Autodesk Inventor part; units mm, degrees
ref_plane "YZ Plane" through (0, 0, 0) normal (1, 0, 0) x (0, 1, 0)
ref_plane "XZ Plane" through (0, 0, 0) normal (0, 1, 0) x (-1, 0, 0)
ref_plane "XY Plane" through (0, 0, 0) normal (0, 0, 1) x (1, 0, 0)
sketch "Sketch1" plane through (0, 0, 0) normal (0, 0, 1) x (1, 0, 0)
  line L0 (-4.1767, 5.9085) -> (6.2233, 5.9085)
  line L1 (6.2233, 5.9085) -> (6.2233, -7.1915)
  line L2 (6.2233, -7.1915) -> (-4.1767, -7.1915)
  line L3 (-4.1767, -7.1915) -> (-4.1767, 5.9085)
  point P0 (0, 0)
  dimension "d0" = 10.4
  dimension "d1" = 13.1
extrude "Extrusion1" add sketch "Sketch1" along normal blind 2
sketch "Sketch2" plane through (0, 0, 2) normal (0, 0, 1) x (1, 0, 0)
  line L0 (-4.1767, -7.1915) -> (6.2233, -7.1915)
  line L1 (6.2233, -7.1915) -> (6.2233, 5.9085)
  line L2 (6.2233, 5.9085) -> (-4.1767, 5.9085)
  line L3 (-4.1767, 5.9085) -> (-4.1767, -7.1915)
  line L4 (6.2233, 5.9085) -> (-4.1767, 5.9085)
  line L5 (1.0233, 5.9085) -> (1.0233, -7.1915)
  line L6 (-4.1767, -7.1915) -> (6.2233, -7.1915)
  line L7 (6.2233, -7.1915) -> (6.2233, 5.9085)
  line L8 (6.2233, -0.6415) -> (-4.1767, -0.6415)
  line L9 (-4.1767, 5.9085) -> (-4.1767, -7.1915)
  line L10 (1.0233, -5.4195) -> (-3.5655, -5.4195)
  line L11 (-3.5655, -5.4195) -> (-3.5655, -2.8116)
  line L12 (-3.5655, -2.8116) -> (1.0233, -2.8116)
  line L13 (1.0233, -2.8116) -> (1.0233, -5.4195)
  point P0 (0, 0)
extrude "Extrusion2" add sketch "Sketch2" along normal blind 1.5 contours L10 L11 L12 L5
sketch "Sketch3" plane through (-3.5655, -2.8116, 2) normal (0, 1, 0) x (1, 0, 0)
  line L0 (0, 0) -> (4.5888, 0)
  line L1 (0, 0) -> (0, -1.5)
  line L2 (4.5888, -1.5) -> (0, -1.5)
  line L3 (4.5888, 0) -> (4.5888, -1.5)
  line L4 (4.5888, -1.5) -> (0, -1.5)
  line L5 (0, 0) -> (0, -1.5)
  line L6 (0, -1.5) -> (-10.2377, -47.6792)
  line L7 (4.5888, -1.5) -> (14.8265, -47.6792)
  arc A0 (-10.2377, -47.6792) -> (14.8265, -47.6792) centre (2.2944, 8.8493) ccw
  line L8 (0, -1.5) -> (4.5888, -1.5)
  point P0 (3.5655, 2)
properties part number "tof"
Can you work these out from the model? Positions are in its coordinate system, mm. A direction names the side the tool comes from. Round coordinates to 2 decimals unless told otherwise and drop trailing zeros. Loops run counter-clockwise (first coordinate to the right, second up) from the corner with the lowest first, then second, coordinate; pieces in that order, holes last. Notation, with made-up numbers: (37, -30) - (41, -30) arc R15 cw to (41, -9) - close; hole circle Ø2 at (-36.5, 27). An arc over 180 degrees is marked (long way). Use CSV: the item, a comma, the result in double quotes. Start each with the question number.
1) If we section it at A-A on y = -5.25: Write out the boundary of the cut face in (x, z).
2) Please list where these lines run through material, in increasing order: probe 1 along Z at (x, y) = (4.5, 0.75); probe 2 along Y at (x, z) = (-2.25, 3.25); probe 3 along X at (y, z) = (-4.25, 2.1). Write a range as [from, to].
3) If we section it at B-B on x = -1.75: Write out the boundary of the cut face in (y, z).
4) For faces 1 (the flat face through (-1, -5.42, 3)), 2 (the flat face through (-4.177, -1, 1)), 3 (the flat face through (1.023, -4, 3)), 4 (the flat face through (-1, -2.812, 3)), 5 (the flat face through (-3.566, -4, 3)), which set-ups out of +Z, -Z, +X, -X, +Y, -Y let a thin tool reach every point of the face, with its end or its side?
5) If we section it at C-C on z = 2.7: Write out the boundary of the cut face in (x, y), plus the area to 3 significant figures.
6) If we section it at D-D on y = 2: Write out the boundary of the cut face in (x, z), plus the area to 3 significant figures.
7) For pin 1 Ø5 at (x, y) = (-0.5, 3.5) entering from +Z; pin 2 Ø0.8 at (y, z) = (-4, 2.5) entering from +X, each with a flat end and sliding along its axis, tell me the tip position at first contact or that it passes through.
Geometry results:
1,outline,"(-4.18, 0) - (6.22, 0) - (6.22, 2) - (1.02, 2) - (1.02, 3.5) - (-3.57, 3.5) - (-3.57, 2) - (-4.18, 2) - close"
2,probe 1,"z = [0, 2]"
2,probe 2,"y = [-5.42, -2.81]"
2,probe 3,"x = [-3.57, 1.02]"
3,outline,"(-7.19, 0) - (5.91, 0) - (5.91, 2) - (-2.81, 2) - (-2.81, 3.5) - (-5.42, 3.5) - (-5.42, 2) - (-7.19, 2) - close"
4,face 1,"+Z, +X, -X, -Y"
4,face 2,"+Z, -Z, -X, +Y, -Y"
4,face 3,"+Z, +X, +Y, -Y"
4,face 4,"+Z, +X, -X, +Y"
4,face 5,"+Z, -X, +Y, -Y"
5,outline,"(-3.57, -5.42) - (1.02, -5.42) - (1.02, -2.81) - (-3.57, -2.81) - close"
5,area,"12.0 mm2"
6,outline,"(-4.18, 0) - (6.22, 0) - (6.22, 2) - (-4.18, 2) - close"
6,area,"20.8 mm2"
7,pin 1,"stops at z = 2"
7,pin 2,"stops at x = 1.02"
